Could you check a few things on this model? Use its own coordinates, in mm. Round coordinates to 2 decimals unless told otherwise and drop trailing zeros. Loops run counter-clockwise (first coordinate to the right, second up) from the corner with the lowest first, then second, coordinate; pieces in that order, holes last. Notation, with made-up numbers: M -2.5,54 L 10.5,54 A16 cw 10.5,77 Z; hole C 34.5,17.5 d5. An arc over 180 degrees is marked long. Answer in a Markdown table with one row per item.
```python
from build123d import *

# Parameters (mm, degrees)
SKETCH1_R           = 50.8
BOSS_EXTRUDE1_DEPTH = 50.8
SKETCH3_R           = 1.190625
BOSS_EXTRUDE3_DEPTH = 1.588262


with BuildPart() as part:
    # Sketch1 → Boss-Extrude1 (new body)
    with BuildSketch(Plane(origin=(0, 0, 0), x_dir=(1, 0, 0), z_dir=(0, 1, 0))):
        Circle(SKETCH1_R)
    extrude(amount=BOSS_EXTRUDE1_DEPTH)

    # Sketch3 → Boss-Extrude3 (add)
    with BuildSketch(Plane(origin=(0, 50.8, 0), x_dir=(1, 0, 0), z_dir=(0, 1, 0))):
        with Locations((28.575, 31.75)):
            Circle(SKETCH3_R)
        with Locations((-28.575, 31.75)):
            Circle(SKETCH3_R)
    extrude(amount=BOSS_EXTRUDE3_DEPTH)


solid = part.part
```
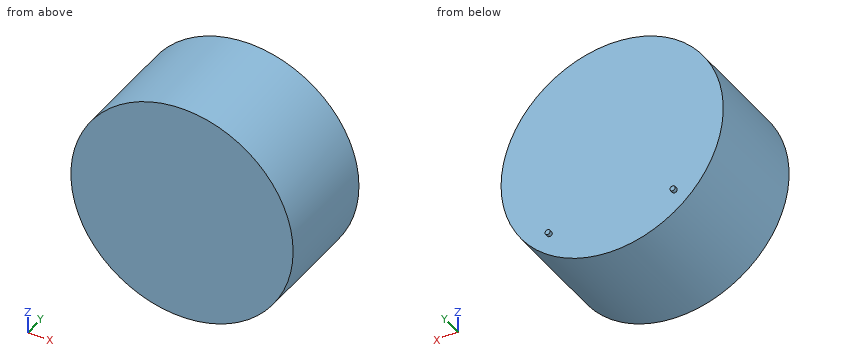
1) Will these pins go through, and if not, where does the flat tip stop? P1, Ø6, axis at x = 22.5, z = -17, coming from the +Y side; P2, Ø6, axis at x = -16, y = 40.5, coming from the +Z side; P3, Ø1, axis at y = 43.5, z = 28.5, coming from the +X side.
Computed:
| item | result |
|---|---|
| P1 | stops at y = 50.8 |
| P2 | stops at z = 49.11 |
| P3 | stops at x = 42.39 |
2) I want a section at A-A, the plane y = 47. Please give me the cut outline in (x, z), plus the area to 3 significant figures.
Computed:
| item | result |
|---|---|
| outline | C 0,0 d101.6 |
| area | 8,110 mm² |
3) I want a section at C-C, the plane x = 0. Please give me the cut outline in (y, z).
Computed:
| item | result |
|---|---|
| outline | M 0,-50.8 L 50.8,-50.8 L 50.8,50.8 L 0,50.8 Z |
4) I need wall thicknesses on line 1 (Y direction, x = -6.5, z = 18.5); line 2 (X direction, y = 34, z = 1); line 3 (X direction, y = 23.5, z = 13.5). Which ranges of each line are inside material? Lowest first, please.
Computed:
| item | result |
|---|---|
| line 1 | y = 0 to 50.8 |
| line 2 | x = -50.79 to 50.79 |
| line 3 | x = -48.97 to 48.97 |
5) I want a section at B-B, the plane z = 0. Please give me the cut outline in (x, y).
Computed:
| item | result |
|---|---|
| outline | M -50.8,0 L 50.8,0 L 50.8,50.8 L -50.8,50.8 Z |
